Could you check a few things on this model? Use its own coordinates, in mm. Give positions to 0.01 mm unless a question says otherwise; leave off trailing zeros. Write each loop counter-clockwise with the first axis right and the second up, starting at its lowest first coordinate (ties: lowest second). Pieces come first, ordered by that corner, then holes. Notation, with made-up numbers: (-24, 59.5) - (4, 59.5) arc R21 ccw to (4, 69.5) - close; hole circle Ø2 at (-37.5, -18.5). An arc over 180 degrees is marked (long way). Use one line per item in the form item = value.
Autodesk Inventor part; units mm, degrees
ref_plane "YZ Plane" through (0, 0, 0) normal (1, 0, 0) x (0, 1, 0)
ref_plane "XZ Plane" through (0, 0, 0) normal (0, 1, 0) x (-1, 0, 0)
ref_plane "XY Plane" through (0, 0, 0) normal (0, 0, 1) x (1, 0, 0)
sketch "Sketch1" plane through (0, 0, 0) normal (0, 0, 1) x (1, 0, 0)
  circle A0 centre (0, 0) radius 8
  dimension "d0" = 16
extrude "Extrusion1" add sketch "Sketch1" along normal blind 100
sketch "Sketch2" plane through (0, 0, 100) normal (0, 0, 1) x (1, 0, 0)
  circle A0 centre (0, 0) radius 14
  dimension "d3" = 28
extrude "Extrusion2" add sketch "Sketch2" along normal blind 10
sketch "Sketch3" plane through (0, 0, 0) normal (0, 0, -1) x (-1, 0, 0)
  circle A0 centre (0, 0) radius 8
extrude "Extrusion3" cut sketch "Sketch3" against normal blind 8
sketch "Sketch4" plane through (0, 0, 8) normal (0, 0, -1) x (-1, 0, 0)
  circle A0 centre (0, 0) radius 8
extrude "Extrusion4" cut sketch "Sketch4" against normal blind 3
sketch "Sketch5" plane through (0, 0, 11) normal (0, 0, -1) x (-1, 0, 0)
  point P0 (0, 0)
sketch "Sketch6" plane through (0, 0, 100) normal (0, 0, -1) x (-1, 0, 0)
  circle A0 centre (0, 0) radius 14
extrude "Extrusion5" add sketch "Sketch6" along normal blind 89
sketch "Sketch7" plane through (0, 0, 11) normal (0, 0, -1) x (-1, 0, 0)
  circle A0 centre (0, 0) radius 4
  dimension "d12" = 8
extrude "Extrusion6" cut sketch "Sketch7" against normal blind 100
properties part number "roll"
1. If we mould it in two halves opening along Y, with no side actions, what happens to faces 1 (the face through (0.867, -3.905, 59.807)), 2 (the face through (3, -3, 110))? For each: pulls with the +Y half, pulls with the -Y half, needs draft (parallel to the pull), parting line crosses it, or undercut.
Response values:
face_1 = undercut
face_2 = needs draft
2. If I drill on line 1 (Y direction, x = 0, z = 82); line 2 (Y direction, x = 2.75, z = 39); line 3 (X direction, y = -2.5, z = 99.5), over which ranges is the centre line in solid material (lowest first)? Write a range as from..to.
Response values:
line_1 = -14..-4, 4..14
line_2 = -13.73..-2.9, 2.9..13.73
line_3 = -13.77..-3.12, 3.12..13.77
3. Imagine slicing it at D-D, the plane x = 10.75. List the corners of the cut face in (y, z) for me.
Response values:
outline = (-8.97, 11) - (8.97, 11) - (8.97, 110) - (-8.97, 110) - close
4. For pin 1 (2 mm diameter, centred on y = -6.5, z = 98, fed in from +X); pin 2 (10 mm diameter, centred on y = 6.5, z = 91.5, fed in from -X); pin 3 (10 mm diameter, centred on x = -8.5, z = 84.5, fed in from -Y), each with a flat end and sliding along its axis, tell me the tip position at first contact or that it passes through.
Response values:
pin_1 = 12.87
pin_2 = -13.92
pin_3 = -13.56
5. Imagine slicing it at A-A, the plane x = 0. List the corners of the cut face in (y, z) for me, and give its area (3 significant figures).
Response values:
outline = (-14, 11) - (-4, 11) - (-4, 110) - (-14, 110) - close; (4, 11) - (14, 11) - (14, 110) - (4, 110) - close
area = 1,980 mm²
6. Imagine slicing it at C-C, the plane z = 56. List the corners of the cut face in (x, y) for me, and give its area (3 significant figures).
Response values:
outline = circle Ø28 at (0, 0); hole circle Ø8 at (0, 0)
area = 565 mm²
